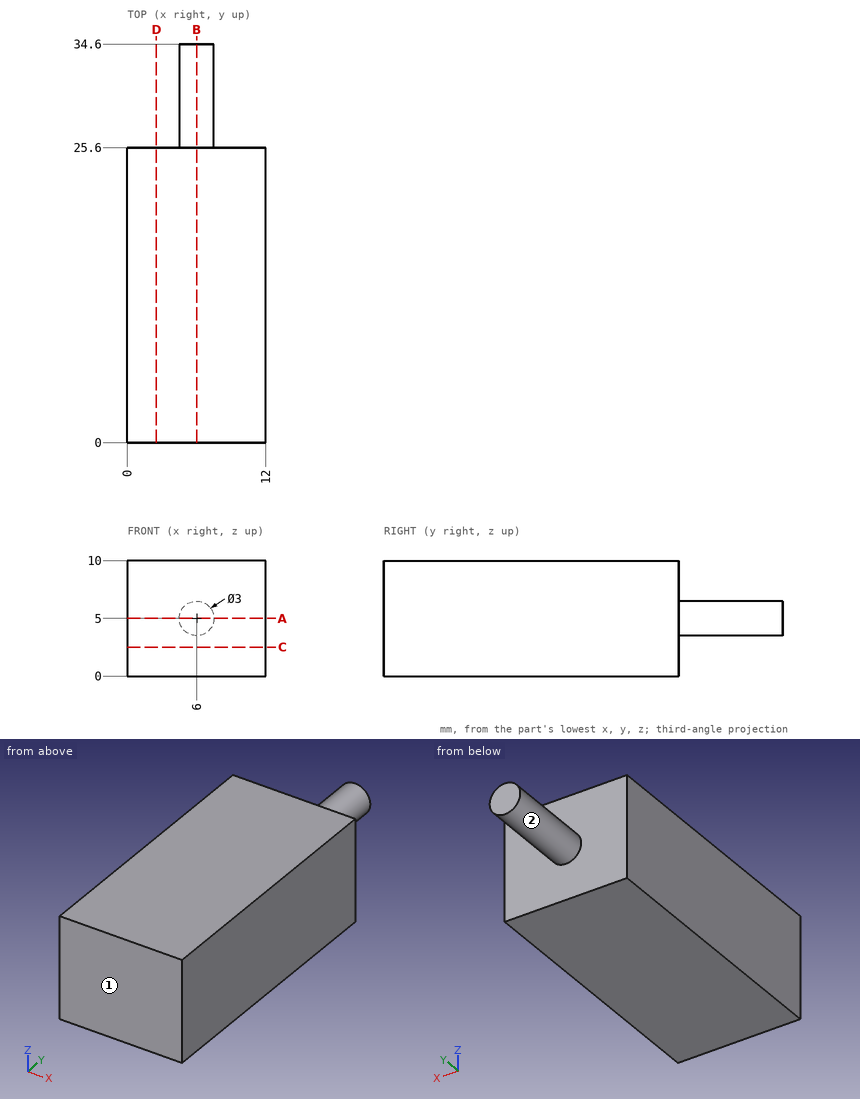
The figure shows three views and two pictorial views of one solid part (mm, origin at its lowest corner). Answer the questions. A direction names the side the tool comes from. Coordinates: 2 decimals unless noted, no trailing zeros. Loops run counter-clockwise (first coordinate to the right, second up) from the corner with the lowest first, then second, coordinate; pieces in that order, holes last. Notation, with made-up numbers: (88.5, 36.5) -> (136.5, 36.5) arc R9 cw to (136.5, 52.5) -> close; hole circle Ø8 at (-14.75, 50). An arc over 180 degrees is marked (long way). Return JSON: item names as keys, results as strings. Group by question number.
(1) A cutting plane is placed at C-C on z = 2.5. Write down the section's boundary in (x, y).
(2) A cutting plane is placed at D-D on x = 2.5. Write down the section's boundary in (y, z).
(3) A cutting plane is placed at A-A on z = 5. Write down the section's boundary in (x, y).
(4) A cutting plane is placed at B-B on x = 6. Write down the section's boundary in (y, z).
(5) Which of the six approach directions +Z, -Z, +X, -X, +Y, -Y give full straight-line access (tool end or side, diameter ignored) to the marked faces 1 and 2?
(6) Find the intervals of material crossed by probe 1 along Y at (x, z) = (1.5, 3); probe 2 along Z at (x, y) = (6, 33); probe 3 along X at (y, z) = (27, 5), in increasing order. Write a range as from..to.
The answers:
{
 "1": {"outline": "(0, 0) -> (12, 0) -> (12, 25.6) -> (0, 25.6) -> close"},
 "2": {"outline": "(0, 0) -> (25.6, 0) -> (25.6, 10) -> (0, 10) -> close"},
 "3": {"outline": "(0, 0) -> (12, 0) -> (12, 25.6) -> (7.5, 25.6) -> (7.5, 34.6) -> (4.5, 34.6) -> (4.5, 25.6) -> (0, 25.6) -> close"},
 "4": {"outline": "(0, 0) -> (25.6, 0) -> (25.6, 3.5) -> (34.6, 3.5) -> (34.6, 6.5) -> (25.6, 6.5) -> (25.6, 10) -> (0, 10) -> close"},
 "5": {"face 1": "+Z, -Z, +X, -X, -Y", "face 2": "+Y"},
 "6": {"probe 1": "y = 0..25.6", "probe 2": "z = 3.5..6.5", "probe 3": "x = 4.5..7.5"}
}
